```python
from build123d import *

# Parameters (mm, degrees)
F1_DEPTH  = 6
F2_W      = 10
F2_H      = 32
F3_DEPTH  = 22
F4_W      = 2
F4_H      = 4.2
F5_DEPTH  = 18
F6_R      = 2
F10_DEPTH = 25
F13_DEPTH = 25
F14_R     = 5
F15_R     = 1
F16_R     = 1


with BuildPart() as f1:
    # F0 (on Top) → F1 (new body)
    with BuildSketch(Plane.XY):
        with BuildLine():
            ThreePointArc((0, -16), (11.313708499, -11.313708499), (16, 0))
            ThreePointArc((16, 0), (11.313708499, 11.313708499), (0, 16))
            Line((0, 16), (0, -16))
        make_face()
        with BuildLine():
            Line((0, -16), (0, 16))
            ThreePointArc((0, 16), (-16, 0), (0, -16))
        make_face()
        with BuildLine():
            ThreePointArc((0, -16), (-16, 0), (0, 16))
            Line((0, 16), (-40.5, 16))
            Line((-40.5, 16), (-40.5, -16))
            Line((-40.5, -16), (0, -16))
        make_face()
    extrude(amount=F1_DEPTH)

    # F2 (on Top) → F3 (join)
    with BuildSketch(Plane.XY):
        with Locations((-35.5, 0)):
            Rectangle(F2_W, F2_H)
    extrude(amount=F3_DEPTH)

    # F4 (on Top) → F5 (cut)
    with BuildSketch(Plane.XY):
        Polygon((-34.9, 13), (-38.5, 13), (-38.5, 11.1), (-38.5, 6.9), (-38.5, 5), (-34.9, 5), align=None)
        with Locations((-39.5, 9)):
            Rectangle(F4_W, F4_H)
    extrude(amount=F5_DEPTH, mode=Mode.SUBTRACT)

    # F6
    f6_edges = [f1.edges().sort_by_distance(p)[0] for p in [
        (-39.5, 6.9, 18),
        (-39.5, 11.1, 18),
    ]]
    fillet(f6_edges, radius=F6_R)

    # F7: F1 across plane


with BuildPart() as f1_1:
    add(f1.part)
    add(f1.part.mirror(Plane.XZ), mode=Mode.INTERSECT)

    # F9 (on offset) → F10 (cut)
    with BuildSketch(Plane.XY.offset(6)):
        Polygon((-30.5, 13), (-38.5, 13), (-38.5, 5), (-34.9, 5), (-34.9, -5), (-38.5, -5), (-38.5, -13), (-30.5, -13), align=None)
    extrude(amount=F10_DEPTH, mode=Mode.SUBTRACT)

    # F12 (on face) → F13 (cut)
    with BuildSketch(Plane.XY):
        with BuildLine():
            Line((-3.3763886032, -5.2), (3.3763886032, -5.2))
            ThreePointArc((3.3763886032, -5.2), (6.2, 0), (3.3763886032, 5.2))
            Line((3.3763886032, 5.2), (-3.3763886032, 5.2))
            ThreePointArc((-3.3763886032, 5.2), (-6.2, 0), (-3.3763886032, -5.2))
        make_face()
    extrude(amount=F13_DEPTH, mode=Mode.SUBTRACT)

    # F14
    f14_edges = [f1_1.edges().sort_by_distance(p)[0] for p in [
        (-35.5, 16, 22),
        (-35.5, -16, 22),
    ]]
    fillet(f14_edges, radius=F14_R)

    # F15
    f15_edges = [f1_1.edges().sort_by_distance(p)[0] for p in [
        (-15.25, 16, 6),
        (16, 0, 6),
        (-15.25, -16, 6),
        (-30.5, -16, 11.5),
        (-30.5, 16, 11.5),
    ]]
    fillet(f15_edges, radius=F15_R)

    # F16
    f16_edges = [f1_1.edges().sort_by_distance(p)[0] for p in [
        (-20.25, 16, 0),
        (-40.5, 0, 0),
        (-40.5, 13.55, 0),
        (-40.5, -13.55, 0),
    ]]
    fillet(f16_edges, radius=F16_R)


solid = f1_1.part
```
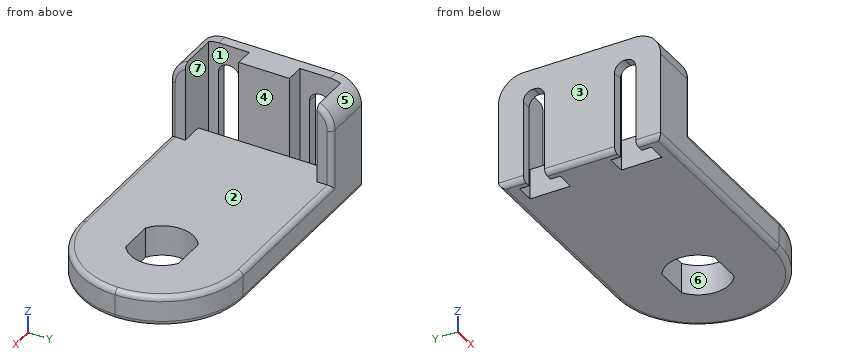
Verification items for the finished model (mm, model axes). Face numbers are marked on the shaded views. A direction names the side the tool comes from. Coordinates: 2 decimals unless noted, no trailing zeros. Order: outer loops, then holes, each group sorted by start corner. A loop starts at its lowest first (then second) coordinate and runs counter-clockwise, first axis right, second up. Notation, with made-up numbers: (-33, 12) -> (11, 12) arc R31 ccw to (11, 47) -> close; hole circle Ø10 at (41.5, -4.5). An arc over 180 degrees is marked (long way). Answer as CSV lines item,"result". Start each with the question number.
1) Release check for a two-part mould opening along X. For the marked faces 1, 2 and 3 record: released by +X, released by -X, zero draft, split by the parting line, or undercut.
2) Material ranges on L1, parallel to X at y = 1, z = 20.75; L2, parallel to X at y = 13.5, z = 12; L3, parallel to Z at x = 4.5, y = 10, recorded low to high. Write a range as [from, to].
3) Cross-section at B-B, the plane x = -34. Record the boundary of the cut face in (y, z), then the cut area to 3 significant figures.
4) Cross-section at C-C, the plane x = -26.5. Record the boundary of the cut face in (y, z), then the cut area to 3 significant figures.
5) Gauge pin test, flat ends, axial feed: pin 1 Ø6.5 at (y, z) = (-11, 3) entering from -X; pin 2 Ø5 at (y, z) = (-2.5, 9.5) entering from +X; pin 3 Ø4 at (x, z) = (6, 2.5) entering from +Y; pin 4 Ø1 at (y, z) = (-9, 3.5) entering from -X. Record the tip position at first contact, or that the pin passes through.
6) Set-up check for the marked faces 4, 5, 6 and 7: record each of +Z, -Z, +X, -X, +Y, -Y from which the full face is reachable in a straight line by a thin tool's end or side.
7) Cross-section at A-A, the plane z = 8.75. Record the boundary of the cut face in (x, y), then the cut area to 3 significant figures.
Conclusion:
1,face 1,"undercut"
1,face 2,"zero draft"
1,face 3,"released by -X"
2,L1,"x = [-40.5, -34.9]"
2,L2,"x = [-40.5, -30.5]"
2,L3,"z = [0, 6]"
3,outline,"(-16, 1) arc R1 ccw to (-15, 0) -> (15, 0) arc R1 ccw to (16, 1) -> (16, 17) arc R5 ccw to (13, 21.58) -> (13, 6) -> (-13, 6) -> (-13, 21.58) arc R5 ccw to (-16, 17) -> close"
3,area,"277 mm²"
4,outline,"(-16, 1) arc R1 ccw to (-15, 0) -> (15, 0) arc R1 ccw to (16, 1) -> (16, 5) arc R1 ccw to (15, 6) -> (-15, 6) arc R1 ccw to (-16, 5) -> close"
4,area,"191 mm²"
5,pin 1,"stops at x = -40.5"
5,pin 2,"stops at x = -34.9"
5,pin 3,"stops at y = 15.49"
5,pin 4,"stops at x = -34.9"
6,face 4,"+Z, +X"
6,face 5,"+Z, +X, -X, +Y"
6,face 6,"+Z, -Z"
6,face 7,"+Z"
7,outline,"(-40.5, -16) -> (-31.5, -16) arc R1 ccw to (-30.5, -15) -> (-30.5, -13) -> (-38.5, -13) -> (-38.5, -11.1) -> (-40.5, -11.1) -> close; (-40.5, -6.9) -> (-38.5, -6.9) -> (-38.5, -5) -> (-34.9, -5) -> (-34.9, 5) -> (-38.5, 5) -> (-38.5, 6.9) -> (-40.5, 6.9) -> close; (-40.5, 11.1) -> (-38.5, 11.1) -> (-38.5, 13) -> (-30.5, 13) -> (-30.5, 15) arc R1 ccw to (-31.5, 16) -> (-40.5, 16) -> close"
7,area,"131 mm²"
